```python
from build123d import *

# Parameters (mm, degrees)
SKETCH1_W            = 45
SKETCH1_H            = 45
SKETCH1_R            = 2
BOSS_EXTRUDE1_DEPTH  = 25
SKETCH2_R            = 1.65
SKETCH2_R_2          = 11
CUT_EXTRUDE1_DEPTH   = 25
SKETCH3_R            = 2.9
CUT_EXTRUDE2_DEPTH   = 3
CHAMFER1_SIZE        = 2
SKETCH4_R            = 18.15
CUT_EXTRUDE3_DEPTH   = 18.5
SKETCH_4_R           = 2
CUT_EXTRUDE_10_DEPTH = 4


with BuildPart() as part:
    # Sketch1 → Boss-Extrude1 (new body)
    with BuildSketch(Plane.XY):
        Rectangle(SKETCH1_W, SKETCH1_H)
        with Locations((-17.5, 17.5)):
            Circle(SKETCH1_R, mode=Mode.SUBTRACT)
        with Locations((17.5, 17.5)):
            Circle(SKETCH1_R, mode=Mode.SUBTRACT)
        with Locations((17.5, -17.5)):
            Circle(SKETCH1_R, mode=Mode.SUBTRACT)
        with Locations((-17.5, -17.5)):
            Circle(SKETCH1_R, mode=Mode.SUBTRACT)
    extrude(amount=BOSS_EXTRUDE1_DEPTH)

    # Sketch2 → Cut-Extrude1 (cut)
    with BuildSketch(Plane.XY.offset(25)):
        with Locations((9.899494937, 9.899494937)):
            Circle(SKETCH2_R)
        with Locations((9.899494937, -9.899494937)):
            Circle(SKETCH2_R)
        with Locations((-9.899494937, -9.899494937)):
            Circle(SKETCH2_R)
        with Locations((-9.899494937, 9.899494937)):
            Circle(SKETCH2_R)
        Circle(SKETCH2_R_2)
    extrude(amount=-CUT_EXTRUDE1_DEPTH, mode=Mode.SUBTRACT)

    # Sketch3 → Cut-Extrude2 (cut)
    with BuildSketch(Plane.XY.offset(25)):
        with Locations((9.899494937, 9.899494937)):
            Circle(SKETCH3_R)
        with Locations((9.899494937, -9.899494937)):
            Circle(SKETCH3_R)
        with Locations((-9.899494937, -9.899494937)):
            Circle(SKETCH3_R)
        with Locations((-9.899494937, 9.899494937)):
            Circle(SKETCH3_R)
    extrude(amount=-CUT_EXTRUDE2_DEPTH, mode=Mode.SUBTRACT)

    # Chamfer1
    chamfer1_edges = [part.edges().sort_by_distance(p)[0] for p in [
        (22.5, -22.5, 12.5),
        (-22.5, -22.5, 12.5),
        (-22.5, 22.5, 12.5),
        (22.5, 22.5, 12.5),
    ]]
    chamfer(chamfer1_edges, length=CHAMFER1_SIZE)

    # Sketch4 → Cut-Extrude3 (cut)
    with BuildSketch(Plane(origin=(0, 0, 0), x_dir=(-1, 0, 0), z_dir=(0, 0, -1))):
        Circle(SKETCH4_R)
    extrude(amount=-CUT_EXTRUDE3_DEPTH, mode=Mode.SUBTRACT)

    # 草图4 → 切除-拉伸10 (cut)
    with BuildSketch(Plane(origin=(0, 0, 0), x_dir=(-1, 0, 0), z_dir=(0, 0, -1))):
        Polygon((13.9, 19.578460969), (13.9, 15.421539031), (17.5, 13.343078062), (21.1, 15.421539031), (21.1, 19.578460969), (17.5, 21.656921938), align=None)
        with Locations((17.5, 17.5)):
            Circle(SKETCH_4_R, mode=Mode.SUBTRACT)
        Polygon((-21.1, 19.578460969), (-21.1, 15.421539031), (-17.5, 13.343078062), (-13.9, 15.421539031), (-13.9, 19.578460969), (-17.5, 21.656921938), align=None)
        with Locations((-17.5, 17.5)):
            Circle(SKETCH_4_R, mode=Mode.SUBTRACT)
        Polygon((-21.1, -15.421539031), (-21.1, -19.578460969), (-17.5, -21.656921938), (-13.9, -19.578460969), (-13.9, -15.421539031), (-17.5, -13.343078062), align=None)
        with Locations((-17.5, -17.5)):
            Circle(SKETCH_4_R, mode=Mode.SUBTRACT)
        Polygon((13.9, -15.421539031), (13.9, -19.578460969), (17.5, -21.656921938), (21.1, -19.578460969), (21.1, -15.421539031), (17.5, -13.343078062), align=None)
        with Locations((17.5, -17.5)):
            Circle(SKETCH_4_R, mode=Mode.SUBTRACT)
    extrude(amount=-CUT_EXTRUDE_10_DEPTH, mode=Mode.SUBTRACT)


solid = part.part
```
For this review, take the finished solid that the model builds, in its own axes (mm). A direction names the side the tool comes from. Coordinates: 2 decimals unless noted, no trailing zeros. Write each loop counter-clockwise with the first axis right and the second up, starting at its lowest first coordinate (ties: lowest second). Pieces come first, ordered by that corner, then holes. Notation, with made-up numbers: (85.5, 38.25) - (118.5, 38.25) arc R7 ccw to (118.5, 47.25) - close; hole circle Ø8 at (-37, -30). An arc over 180 degrees is marked (long way). Put each result on its own line as item: value.
1. Add section B-B, the plane x = -3.5. Give the boundary of the cut face in (y, z).
Values found:
outline: (-22.5, 0) - (-17.81, 0) - (-17.81, 18.5) - (-10.43, 18.5) - (-10.43, 25) - (-22.5, 25) - close; (10.43, 18.5) - (17.81, 18.5) - (17.81, 0) - (22.5, 0) - (22.5, 25) - (10.43, 25) - close
2. Machinability: for faces 4 (the cylindrical face through (-12, -7.9, 23.5)), 5 (the flat face through (22, 21, 12)), 6 (the flat face through (19.275, -14.368, 1.972)), which of the approach directions +Z, -Z, +X, -X, +Y, -Y give a long, thin tool a straight path to every point of the face, cutting with its end or side? Answer none if there is none.
Values found:
face 4: +Z
face 5: +Z, -Z, +X, +Y
face 6: -Z
3. Mouldability with a two-part tool opening along Y and no side actions: class faces 1 (the flat face through (-15.8, 15.7, 4)), 2 (the flat face through (-21, 22, 12)), 3 (the flat face through (-21, -22, 12)) as released by +Y, released by -Y, zero draft, split by the parting line, or undercut.
Values found:
face 1: undercut
face 2: released by +Y
face 3: released by -Y
4. Add section A-A, the plane y = 0. Give the boundary of the cut face in (x, z), then the cut area to 3 significant figures.
Values found:
outline: (-22.5, 0) - (-18.15, 0) - (-18.15, 18.5) - (-11, 18.5) - (-11, 25) - (-22.5, 25) - close; (11, 18.5) - (18.15, 18.5) - (18.15, 0) - (22.5, 0) - (22.5, 25) - (11, 25) - close
area: 310 mm²
5. Add section D-D, the plane y = -17.5. Give the boundary of the cut face in (x, z).
Values found:
outline: (-22.5, 0) - (-21.1, 0) - (-21.1, 4) - (-19.5, 4) - (-19.5, 25) - (-22.5, 25) - close; (-15.5, 4) - (-13.9, 4) - (-13.9, 0) - (-4.81, 0) - (-4.81, 18.5) - (4.81, 18.5) - (4.81, 0) - (13.9, 0) - (13.9, 4) - (15.5, 4) - (15.5, 25) - (-15.5, 25) - close; (19.5, 4) - (21.1, 4) - (21.1, 0) - (22.5, 0) - (22.5, 25) - (19.5, 25) - close
6. Wall thickness on probe 1 along X at (y, z) = (20.5, 3.75); probe 2 along Y at (x, z) = (-20, 3.25); probe 3 along X at (y, z) = (-8, 23): over which ranges is each line inside the solid? List them lowest first.
Values found:
probe 1: -22.5 to -19.5, -15.5 to 15.5, 19.5 to 22.5
probe 2: -22.5 to -20.21, -14.79 to 14.79, 20.21 to 22.5
probe 3: -22.5 to -12.09, -7.71 to -7.55, 7.55 to 7.71, 12.09 to 22.5
7. For pin 1 (1.5 mm diameter, centred on x = -9, y = 6.5, fed in from -Z); pin 2 (3 mm diameter, centred on x = 17.5, y = 17.5, fed in from -Z); pin 3 (4.5 mm diameter, centred on x = -9.9, y = -9.9, fed in from +Z); pin 4 (3.5 mm diameter, centred on x = 16.5, y = 18.5, fed in from -Z), all flat-tipped, find the tip position at first contact; note any pin that passes through.
Values found:
pin 1: z = 18.5
pin 2: through
pin 3: z = 22
pin 4: z = 4
8. Add section C-C, the plane z = 17.75. Give the boundary of the cut face in (x, y).
Values found:
outline: (-22.5, -20.5) - (-20.5, -22.5) - (20.5, -22.5) - (22.5, -20.5) - (22.5, 20.5) - (20.5, 22.5) - (-20.5, 22.5) - (-22.5, 20.5) - close; hole circle Ø4 at (-17.5, -17.5); hole circle Ø4 at (-17.5, 17.5); hole circle Ø36.3 at (0, 0); hole circle Ø4 at (17.5, -17.5); hole circle Ø4 at (17.5, 17.5)
